Source: CAD feature listing. Evaluate the final solid. Frame: model axes, mm. A direction names the side the tool comes from. Give positions to 0.01 mm unless a question says otherwise; leave off trailing zeros. Order: outer loops, then holes, each group sorted by start corner. A loop starts at its lowest first (then second) coordinate and runs counter-clockwise, first axis right, second up. Notation, with made-up numbers: M 31,37.25 L 42,37.25 A31 ccw 42,66.25 Z; hole C 52.25,78.5 d5. An arc over 180 degrees is marked long. Answer in a Markdown table with one row per item. Add a question column.
(1) Mould query, pull axis X, two halves, no side actions, for faces 1 (the face through (7.65, 10.09, 1.88)), 2 (the face through (-2.5, 10, 8)), 3 (the face through (21, 14.7, 9)). Classes: pulls with the +X half, pulls with the -X half, needs draft (parallel to the pull), parting line crosses it, or undercut.
(2) Set-up query: faces 4 (the face through (-1, 14.7, 9)), 5 (the face through (5, 10, 14)), 6 (the face through (21, 10, 11)), 7 (the face through (21, 10, 4.6)), 8 (the face through (-1, 10, 11)). Return all of +Z, -Z, +X, -X, +Y, -Y with unobstructed straight access to the full face (end or side cutting, diameter ignored); none if empty.
(3) Section query A-A, the plane y = 10. Return loops of the section in (x, z), plus the area to 3 significant figures.
(4) Section query D-D, the plane z = 17.75. Return loops of the section in (x, y).
(5) Section query C-C, the plane z = 9.75. Return loops of the section in (x, y), plus the area to 3 significant figures.
(6) Pin query (flat end, axial travel): P1, Ø1.2, axis at x = 20.5, z = 7, coming from the -Y side; P2, Ø3, axis at x = 11, y = 3.5, coming from the +Z side; P3, Ø4.5, axis at y = 10, z = 17.75, coming from the +X side; P4, Ø2, axis at y = 17, z = 8, coming from the -X side. Return the tip coordinate at first contact, or that it passes through.
(7) Section query B-B, the plane x = 9.75. Return loops of the section in (y, z).
(8) Material intervals for line 1 along X through (y, z) = (13.25, 10.75); line 2 along X through (y, z) = (10.75, 4.5); line 3 along Y through (x, z) = (16, 17.75), sorted ascending.
from build123d import *

# Parameters (mm, degrees)
BOSS_EXTRUDE1_DEPTH = 20
M5_TAPPED_HOLE1_D   = 4.2
SKETCH5_R           = 2.5
CUT_EXTRUDE1_DEPTH  = 38.486664295
BOSS_EXTRUDE2_DEPTH = 2.5


with BuildPart() as part:
    # Sketch1 → Boss-Extrude1 (new body)
    with BuildSketch(Plane(origin=(0, 0, 0), x_dir=(1, 0, 0), z_dir=(0, 1, 0))):
        Polygon((14.5, -25), (19.5, -25), (19.5, 0), (0, 0), (0, -25), (5, -25), (5, -3.7), (14.5, -3.7), align=None)
    extrude(amount=BOSS_EXTRUDE1_DEPTH)

    # M5 Tapped Hole1 (through all)
    with Locations(Plane(origin=(0, 0, 0), x_dir=(-1, 0, 0), z_dir=(0, 0, -1))):
        with Locations((-9.75, 10)):
            Hole(M5_TAPPED_HOLE1_D / 2)

    # Sketch5 → Cut-Extrude1 (cut, through all)
    with BuildSketch(Plane(origin=(19.5, 0, 0), x_dir=(0, 0, -1), z_dir=(1, 0, 0))):
        with Locations((-17.75, 10)):
            Circle(SKETCH5_R)
    extrude(amount=-CUT_EXTRUDE1_DEPTH, mode=Mode.SUBTRACT)

    # Sketch6 → Boss-Extrude2 (add)
    with BuildSketch(Plane(origin=(19.5, 0, 0), x_dir=(0, 0, -1), z_dir=(1, 0, 0))):
        with BuildLine():
            Line((-13.85, 14.7), (-4.6, 14.7))
            Line((-4.6, 14.7), (-4.6, 5.3))
            Line((-4.6, 5.3), (-13.85, 5.3))
            ThreePointArc((-13.85, 5.3), (-10.999489743, 10), (-13.85, 14.7))
        make_face()
    boss_extrude2 = extrude(amount=BOSS_EXTRUDE2_DEPTH)

    # Mirror1: Boss-Extrude2 across plane
    add(boss_extrude2.mirror(Plane(origin=(9.75, 0, 0), x_dir=(0, 0, 1), z_dir=(1, 0, 0))))


solid = part.part
Values follow:
| question | item | result |
|---|---|---|
| 1 | face 1 | undercut |
| 1 | face 2 | pulls with the -X half |
| 1 | face 3 | needs draft |
| 2 | face 4 | +Z, -Z, -X, +Y |
| 2 | face 5 | +Z, +Y, -Y |
| 2 | face 6 | +Z, +X |
| 2 | face 7 | -Z, +X, +Y, -Y |
| 2 | face 8 | +Z, -X |
| 3 | outline | M -2.5,4.6 L 0,4.6 L 0,0 L 7.65,0 L 7.65,3.7 L 5,3.7 L 5,15.25 L 0,15.25 L 0,11 L -2.5,11 Z; M 0,20.25 L 5,20.25 L 5,25 L 0,25 Z; M 11.85,0 L 19.5,0 L 19.5,4.6 L 22,4.6 L 22,11 L 19.5,11 L 19.5,15.25 L 14.5,15.25 L 14.5,3.7 L 11.85,3.7 Z; M 14.5,20.25 L 19.5,20.25 L 19.5,25 L 14.5,25 Z |
| 3 | area | 252 mm² |
| 4 | outline | M 0,0 L 5,0 L 5,7.5 L 0,7.5 Z; M 0,12.5 L 5,12.5 L 5,20 L 0,20 Z; M 14.5,0 L 19.5,0 L 19.5,7.5 L 14.5,7.5 Z; M 14.5,12.5 L 19.5,12.5 L 19.5,20 L 14.5,20 Z |
| 5 | outline | M -2.5,5.3 L 0,5.3 L 0,0 L 5,0 L 5,20 L 0,20 L 0,14.7 L -2.5,14.7 Z; M 14.5,0 L 19.5,0 L 19.5,5.3 L 22,5.3 L 22,14.7 L 19.5,14.7 L 19.5,20 L 14.5,20 Z |
| 5 | area | 247 mm² |
| 6 | P1 | stops at y = 5.3 |
| 6 | P2 | stops at z = 3.7 |
| 6 | P3 | passes through |
| 6 | P4 | stops at x = 0 |
| 7 | outline | M 0,0 L 7.9,0 L 7.9,3.7 L 0,3.7 Z; M 12.1,0 L 20,0 L 20,3.7 L 12.1,3.7 Z |
| 8 | line 1 | x = -2.5 to 5, 14.5 to 22 |
| 8 | line 2 | x = 0 to 5, 14.5 to 19.5 |
| 8 | line 3 | y = 0 to 7.5, 12.5 to 20 |
